Work out the finished part from the listing and answer in its coordinate system (mm). A direction names the side the tool comes from. Round coordinates to 2 decimals unless told otherwise and drop trailing zeros. Loops run counter-clockwise (first coordinate to the right, second up) from the corner with the lowest first, then second, coordinate; pieces in that order, holes last.
Autodesk Fusion 360 part; units mm, degrees
sketch "Sketch2" plane through (0, 30, 0) normal (0, 1, 0) x (-1, 0, 0)
  circle A0 centre (0, 0) radius 3
  circle A1 centre (0, 0) radius 3
ref_plane "WorkPlane1" through (0, 23.5, 0) normal (0, 1, 0) x (-1, 0, 0)
ref_plane "WorkPlane2" through (0, 22.5, 0) normal (0, 1, 0) x (-1, 0, 0)
sketch "Sketch3" plane through (0, 22.5, 0) normal (0, 1, 0) x (1, 0, 0)
  circle A0 centre (0, 0) radius 2.25
  dimension "d12" = 4.5
sketch "Sketch4" plane through (0, 23.5, 0) normal (0, 1, 0) x (1, 0, 0)
  circle A0 centre (0, 0) radius 3
  dimension "d13" = 6
extrude "Extrude2" add sketch "Sketch2" against normal blind 6.5
loft "Loft1" add profiles "Sketch4", "Sketch3" section 1 section 2
extrude "Extrude3" add 1 faces at (-0.1619, 22.5, 0.6982) along direction (0, -1, 0) blind 16.75
ref_plane "WorkPlane3" through (0, 4.75, 0) normal (0, -1, 0) x (0, 0, -1)
sketch "Sketch5" plane through (0, 4.75, 0) normal (0, -1, 0) x (1, 0, 0)
  circle A0 centre (0, 0) radius 3
  dimension "d19" = 6
loft "Loft2" add profiles "Sketch5" section 1 face at (-0.1619, 5.75, 0.6982) section 2
extrude "Extrude4" add 1 faces at (-1.1591, 4.75, 0.5829) along direction (0, -1, 0) blind 5.5
extrude "Extrude5" cut 1 faces at (1.1591, 30, 0.5829) along direction (0, -1, 0) blind 0.75
hole "Hole3" at (0, 29.25, 0) direction (0, -1, 0) diameter 3 depth 5 tip angle 118
hole "Hole4" at (0, -0.75, 0) direction (0, 1, 0) diameter 3 depth 5 tip angle 118
thread "Thread3"
thread "Thread4"
1. Given pin 1 (1 mm diameter, centred on x = 1.5, y = 15.5, fed in from +Z); pin 2 (1 mm diameter, centred on x = -1, y = 8, fed in from +Z); pin 3 (2.5 mm diameter, centred on x = 0, z = 0, fed in from +Y), each flat-ended and moving along its own axis, determine where each tip first touches the part or whether it passes through.
Answer key:
pin 1: stops at z = 2.02
pin 2: stops at z = 2.19
pin 3: stops at y = 24.1
2. Determine the mould class of faces 1 (the face through (-3, 2, 0)), 2 (the face through (-0.29, 14.24, -2.23)), 3 (the face through (1.3, -0.75, -1.3)), 4 (the face through (-1.3, 29.25, -1.3)) for opening direction Y: +Y half, -Y half, draft (parallel to the pull), parting line (faces both ways), or undercut.
Answer key:
face 1: draft
face 2: undercut
face 3: -Y half
face 4: +Y half
3. Which of the six approach directions +Z, -Z, +X, -X, +Y, -Y give full straight-line access (tool end or side, diameter ignored) to faces 5 (the face through (-0.07, 1.78, 1.5)), 6 (the face through (-0.07, 26.72, -1.5)), 7 (the face through (3, 26, 0))?
Answer key:
face 5: -Y
face 6: +Y
face 7: +Y, -Y
4. Consider probe 1 along X at (y, z) = (26.2, 0); probe 2 along X at (y, z) = (22.25, 0). Determine where each line is inside the solid, lowest interval first.
Answer key:
probe 1: x = -3 to -1.5, 1.5 to 3
probe 2: x = -2.25 to 2.25
5. Find section A-A (y = 18.75). Write down the section's boundary in (x, z).
Answer key:
outline: circle Ø4.5 at (0, 0)
